from build123d import *

# Parameters (mm, degrees)
SKETCH1_W           = 53.975
SKETCH1_H           = 31.75
BOSS_EXTRUDE1_DEPTH = 76.2
SHELL1_T            = 5
SKETCH2_W           = 44.45
SKETCH2_H           = 53.975
CUT_EXTRUDE1_DEPTH  = 5
FILLET2_R           = 6.35
SKETCH3_W           = 54.53
SKETCH3_H           = 63.975
SKETCH3_W_2         = 44.45
SKETCH3_H_2         = 53.975
BOSS_EXTRUDE2_DEPTH = 19.05
FILLET5_R           = 3.175
FILLET6_R           = 3.175
SKETCH4_W           = 53.975
SKETCH4_H           = 15.875
BOSS_EXTRUDE3_DEPTH = 25.4
SHELL2_T            = 5
SKETCH5_W           = 15.875
SKETCH5_H           = 53.975
CUT_EXTRUDE2_DEPTH  = 5
SKETCH6_W           = 25.875
SKETCH6_H           = 63.975
SKETCH6_W_2         = 15.875
SKETCH6_H_2         = 53.975
BOSS_EXTRUDE4_DEPTH = 72.0928
SKETCH7_W           = 15.875
SKETCH7_H           = 53.975
CUT_EXTRUDE3_DEPTH  = 5
FILLET7_R           = 44.45
FILLET8_R           = 46.99
FILLET9_R           = 46.99
FILLET10_R          = 48.26
FILLET11_R          = 6.35
FILLET12_R          = 6.35
FILLET13_R          = 19.05
FILLET14_R          = 25.4
FILLET15_R          = 3.175


with BuildPart() as part:
    # Sketch1 → Boss-Extrude1 (new body)
    with BuildSketch(Plane(origin=(0, 0, 0), x_dir=(0, 0, -1), z_dir=(1, 0, 0))):
        with Locations((106.854663617, 0)):
            Rectangle(SKETCH1_W, SKETCH1_H)
    extrude(amount=BOSS_EXTRUDE1_DEPTH)

    # Shell1
    shell1_openings = [part.faces().sort_by_distance(p)[0] for p in [
        (0, 0, -106.854663617),
    ]]
    offset(amount=SHELL1_T, openings=shell1_openings, kind=Kind.INTERSECTION)

    # Sketch2 → Cut-Extrude1 (cut)
    with BuildSketch(Plane(origin=(0, -20.875, 0), x_dir=(-1, 0, 0), z_dir=(0, -1, 0))):
        with Locations((-53.975, 106.854663617)):
            Rectangle(SKETCH2_W, SKETCH2_H)
    extrude(amount=-CUT_EXTRUDE1_DEPTH, mode=Mode.SUBTRACT)

    # Fillet2
    # the kernel refuses this fillet: 6.35 mm, written as the material it takes off along each edge
    with BuildSketch(Plane(origin=(31.75, -15.875, -79.867163617), x_dir=(-1, 0, 0), z_dir=(0, 0, -1))) as fillet2_piece_1:
        with BuildLine():
            CenterArc((6.204836823, -6.35), FILLET2_R, 90, 77.725329785)
            Line((0, -5), (0, 0))
            Line((0, 0), (6.204836823, 0))
        make_face()
    extrude(amount=53.975, mode=Mode.SUBTRACT)

    # Sketch3 → Boss-Extrude2 (add)
    with BuildSketch(Plane.XZ.offset(20.875)):
        with Locations((53.935, -106.854663617)):
            Rectangle(SKETCH3_W, SKETCH3_H)
        with Locations((53.975, -106.854663617)):
            Rectangle(SKETCH3_W_2, SKETCH3_H_2, mode=Mode.SUBTRACT)
    extrude(amount=BOSS_EXTRUDE2_DEPTH)

    # Fillet5
    fillet5_edges = [part.edges().sort_by_distance(p)[0] for p in [
        (26.67, -20.875, -106.854663617),
    ]]
    fillet(fillet5_edges, radius=FILLET5_R)

    # Fillet6
    fillet6_edges = [part.edges().sort_by_distance(p)[0] for p in [
        (26.67, -39.925, -106.854663617),
        (53.935, -39.925, -74.867163617),
    ]]
    fillet(fillet6_edges, radius=FILLET6_R)



with BuildPart() as body_2:
    # Sketch4 → Boss-Extrude3 (new body)
    with BuildSketch(Plane(origin=(0, 0, 0), x_dir=(0, 0, -1), z_dir=(1, 0, 0))):
        with Locations((106.854663617, 105.9053)):
            Rectangle(SKETCH4_W, SKETCH4_H)
    extrude(amount=BOSS_EXTRUDE3_DEPTH)

    # Shell2
    shell2_openings = [body_2.faces().sort_by_distance(p)[0] for p in [
        (0, 105.9053, -106.854663617),
    ]]
    offset(amount=SHELL2_T, openings=shell2_openings, kind=Kind.INTERSECTION)

    # Sketch5 → Cut-Extrude2 (cut)
    with BuildSketch(Plane.XZ.offset(-92.9678)):
        with Locations((17.4625, -106.854663617)):
            Rectangle(SKETCH5_W, SKETCH5_H)
    extrude(amount=-CUT_EXTRUDE2_DEPTH, mode=Mode.SUBTRACT)


with BuildPart() as part_1:
    add(part.part)

    add(body_2.part)  # Boss-Extrude4 merges body 2
    # Sketch6 → Boss-Extrude4 (add)
    with BuildSketch(Plane.XZ.offset(-92.9678)):
        with Locations((17.4625, -106.854663617)):
            Rectangle(SKETCH6_W, SKETCH6_H)
        with Locations((17.4625, -106.854663617)):
            Rectangle(SKETCH6_W_2, SKETCH6_H_2, mode=Mode.SUBTRACT)
    extrude(amount=BOSS_EXTRUDE4_DEPTH)

    # Sketch7 → Cut-Extrude3 (cut)
    with BuildSketch(Plane.XZ.offset(-15.875)):
        with Locations((17.4625, -106.854663617)):
            Rectangle(SKETCH7_W, SKETCH7_H)
    extrude(amount=-CUT_EXTRUDE3_DEPTH, mode=Mode.SUBTRACT)

    # Fillet7
    fillet7_edges = [part_1.edges().sort_by_distance(p)[0] for p in [
        (30.4, 20.875, -106.854663617),
    ]]
    fillet(fillet7_edges, radius=FILLET7_R)

    # Fillet8
    fillet8_edges = [part_1.edges().sort_by_distance(p)[0] for p in [
        (25.4, 15.875, -106.854663617),
    ]]
    fillet(fillet8_edges, radius=FILLET8_R)

    # Fillet9
    fillet9_edges = [part_1.edges().sort_by_distance(p)[0] for p in [
        (76.2, 15.875, -106.854663617),
    ]]
    fillet(fillet9_edges, radius=FILLET9_R)

    # Fillet10
    fillet10_edges = [part_1.edges().sort_by_distance(p)[0] for p in [
        (81.2, 20.875, -106.854663617),
    ]]
    fillet(fillet10_edges, radius=FILLET10_R)

    # Fillet11
    fillet11_edges = [part_1.edges().sort_by_distance(p)[0] for p in [
        (9.525, 15.875, -106.854663617),
    ]]
    fillet(fillet11_edges, radius=FILLET11_R)

    # Fillet12
    fillet12_edges = [part_1.edges().sort_by_distance(p)[0] for p in [
        (9.525, 97.9678, -106.854663617),
    ]]
    fillet(fillet12_edges, radius=FILLET12_R)

    # Fillet13
    fillet13_edges = [part_1.edges().sort_by_distance(p)[0] for p in [
        (25.4, 113.8428, -106.854663617),
    ]]
    fillet(fillet13_edges, radius=FILLET13_R)

    # Fillet14
    fillet14_edges = [part_1.edges().sort_by_distance(p)[0] for p in [
        (30.4, 118.8428, -106.854663617),
    ]]
    fillet(fillet14_edges, radius=FILLET14_R)

    # Fillet15
    fillet15_edges = [part_1.edges().sort_by_distance(p)[0] for p in [
        (81.2, -28.648204314, -138.842163617),
        (30.4, 79.3839, -74.867163617),
        (30.4, 79.3839, -138.842163617),
        (36.975381235, 42.058806641, -138.842163617),
        (36.975381235, 42.058806641, -74.867163617),
        (74.061014659, 7.889029876, -138.842163617),
        (74.061014659, 7.889029876, -74.867163617),
        (2.5, 118.8428, -74.867163617),
        (2.5, 118.8428, -138.842163617),
        (22.960512242, 111.403312242, -138.842163617),
        (22.960512242, 111.403312242, -74.867163617),
        (81.2, -39.925, -108.442163617),
        (81.2, -27.060704314, -74.867163617),
        (81.2, -38.99506403, -75.797099587),
    ]]
    fillet(fillet15_edges, radius=FILLET15_R)


solid = part_1.part
Can you work these out from the model? Positions are in its coordinate system, mm. A direction names the side the tool comes from. Give positions to 0.01 mm unless a question says otherwise; leave off trailing zeros. Loops run counter-clockwise (first coordinate to the right, second up) from the corner with the lowest first, then second, coordinate; pieces in that order, holes last. Notation, with made-up numbers: (-4, 88) - (40, 88) arc R29 cw to (40, 108) - close; hole circle Ø2 at (64.25, 66.5). An arc over 180 degrees is marked (long way). Return JSON: item names as keys, results as strings.
1. We'd pull the mould along Y, two halves only. Please class faces 1 (the face through (2.465, 117.888, -75.773)), 2 (the face through (76.2, -30, -107)), 3 (the face through (4.525, 57, -107)): +Y half, -Y half, draft (parallel to the pull), parting line (faces both ways), or undercut.
Output values:
{"face 1": "+Y half", "face 2": "draft", "face 3": "undercut"}
2. I want a section at B-B on z = -92.5. Give the number of separate pieces and of enclosed holes in the cut face, and give its area (3 significant figures).
Output values:
{"separate pieces": "3", "enclosed holes": "0", "area": "1,730 mm²"}
3. For faces 4 (the face through (30.4, 80, -107)), 5 (the face through (29, 21, -133.842)), 6 (the face through (29.445, 79.581, -75.773)), which set-ups out of +Z, -Z, +X, -X, +Y, -Y let a thin tool reach every point of the face, with its end or its side?
Output values:
{"face 4": "+Z, -Z, +X, +Y", "face 5": "none", "face 6": "+Z, +X, +Y"}
4. If I drill on line 1 (X direction, y = -25, z = -96.5); line 2 (X direction, y = 74.5, z = -96) (3 decimals); line 3 (Z direction, x = 42.5, y = 22.5), over which ranges is the centre line in solid material (lowest first)?
Output values:
{"line 1": "x = 26.67 to 31.75, 76.2 to 81.2", "line 2": "x = 4.525 to 9.525, 25.4 to 30.4", "line 3": "z = -138.84 to -133.84, -79.87 to -74.87"}
5. I want a section at A-A on y = 77. Please give me the cut outline in (x, z) (3 decimals).
Output values:
{"outline": "(4.525, -138.842) - (27.225, -138.842) arc R3.175 ccw to (30.4, -135.667) - (30.4, -78.042) arc R3.175 ccw to (27.225, -74.867) - (4.525, -74.867) - close; hole (9.525, -133.842) - (25.4, -133.842) - (25.4, -79.867) - (9.525, -79.867) - close"}
6. I'm going to push flat-ended pins straight in: pin 1 Ø22.5 at (y, z) = (85.5, -112.5) entering from +X; pin 2 Ø2 at (y, z) = (63, -119.5) entering from +X; pin 3 Ø19 at (y, z) = (74, -117.5) entering from -X (3 decimals). Where does each tip first touch, or does it pass through?
Output values:
{"pin 1": "stops at x = 30.4", "pin 2": "stops at x = 30.52", "pin 3": "stops at x = 4.525"}
